```python
from build123d import *

# Parameters (mm, degrees)
BOSS_EXTRUDE1_DEPTH = 31.75
CUT_EXTRUDE1_DEPTH  = 25.4
FILLET1_R           = 2.54
CUT_EXTRUDE2_DEPTH  = 25.4
SKETCH5_R           = 0.762
CUT_EXTRUDE3_DEPTH  = 266.7


with BuildPart() as part:
    # Sketch1 → Boss-Extrude1 (new body)
    with BuildSketch(Plane(origin=(0, 0, 0), x_dir=(1, 0, 0), z_dir=(0, 1, 0))):
        with BuildLine():
            Line((12.429156122, 80.324059149), (20.977980966, 99.410685113))
            ThreePointArc((20.977980966, 99.410685113), (0, 101.6), (-20.977980966, 99.410685113))
            Line((-20.977980966, 99.410685113), (-12.429156122, 80.324059149))
            ThreePointArc((-12.429156122, 80.324059149), (0, 81.28), (12.429156122, 80.324059149))
        make_face()
    extrude(amount=BOSS_EXTRUDE1_DEPTH)

    # Sketch3 → Cut-Extrude1 (cut)
    with BuildSketch(Plane.XZ):
        with BuildLine():
            Line((-14.041319773, -83.923473707), (-15.916003555, -88.109006667))
            ThreePointArc((-15.916003555, -88.109006667), (0, -89.535), (15.916003555, -88.109006667))
            Line((15.916003555, -88.109006667), (14.041319773, -83.923473707))
            ThreePointArc((14.041319773, -83.923473707), (0, -85.09), (-14.041319773, -83.923473707))
        make_face()
    extrude(amount=-CUT_EXTRUDE1_DEPTH, mode=Mode.SUBTRACT)

    # Fillet1
    fillet1_edges = [part.edges().sort_by_distance(p)[0] for p in [
        (0, 31.75, -81.28),
        (0, 31.75, -101.6),
    ]]
    fillet(fillet1_edges, radius=FILLET1_R)

    # Sketch4 → Cut-Extrude2 (cut)
    with BuildSketch(Plane.XZ):
        with BuildLine():
            Line((-25.786806636, -94.723734325), (-24.259006715, -92.10897401))
            ThreePointArc((-24.259006715, -92.10897401), (10.833808817, -94.63187141), (44.448447191, -84.243088988))
            Line((44.448447191, -84.243088988), (46.527666616, -86.444904305))
            ThreePointArc((46.527666616, -86.444904305), (11.166045621, -97.533915466), (-25.786806636, -94.723734325))
        make_face()
    extrude(amount=-CUT_EXTRUDE2_DEPTH, mode=Mode.SUBTRACT)

    # Sketch5 → Cut-Extrude3 (cut)
    with BuildSketch(Plane.XY):
        with Locations((0, 6.35)):
            Circle(SKETCH5_R)
    extrude(amount=-CUT_EXTRUDE3_DEPTH, mode=Mode.SUBTRACT)


solid = part.part
```
Here's how the part is built. I have some questions about the finished solid (model axes, mm). A direction names the side the tool comes from. Round coordinates to 2 decimals unless told otherwise and drop trailing zeros. Order: outer loops, then holes, each group sorted by start corner. A loop starts at its lowest first (then second) coordinate and runs counter-clockwise, first axis right, second up. Notation, with made-up numbers: M 4.25,-19 L 24.25,-19 A20 cw 24.25,15 Z; hole C 60,-28 d8. An arc over 180 degrees is marked long. Answer as CSV lines item,"result".
Item 1: For pin 1 (1.5 mm diameter, centred on y = 24, z = -84.5, fed in from +X); pin 2 (2.5 mm diameter, centred on x = 0, y = 6.35, fed in from +Z); pin 3 (2 mm diameter, centred on x = 14.5, z = -86, fed in from -Y), each with a flat end and sliding along its axis, tell me the tip position at first contact or that it passes through.
From the geometry:
pin 1,"x = 14.04"
pin 2,"z = -81.27"
pin 3,"y = 25.4"
Item 2: Imagine slicing it at C-C on y = 6.35. List the corners of the cut face in (x, z) for me (3 decimals).
From the geometry:
outline,"M -20.978,-99.411 A101.6 ccw -0.762,-101.597 L -0.762,-98.168 A98.171 cw -19.543,-96.206 Z; M -18.318,-93.472 A95.25 ccw -0.762,-95.247 L -0.762,-89.532 A89.535 cw -15.916,-88.109 Z; M -14.041,-83.923 A85.09 ccw -0.762,-85.087 L -0.762,-81.276 A81.28 cw -12.429,-80.324 Z; M 0.762,-101.597 A101.6 ccw 20.978,-99.411 L 19.543,-96.206 A98.171 cw 0.762,-98.168 Z; M 0.762,-95.247 A95.25 ccw 18.318,-93.472 L 15.916,-88.109 A89.535 cw 0.762,-89.532 Z; M 0.762,-85.087 A85.09 ccw 14.041,-83.923 L 12.429,-80.324 A81.28 cw 0.762,-81.276 Z"
Item 3: Please list where these lines run through material, in increasing order: L1, parallel to Z at x = -1, y = 16; L2, parallel to Z at x = -11.5, y = 13; L3, parallel to Y at x = 0, z = -84.25. Write a range as [from, to].
From the geometry:
L1,"[-101.6, -98.17], [-95.24, -89.53], [-85.08, -81.27]"
L2,"[-100.95, -97.5], [-94.55, -88.79], [-84.31, -80.46]"
L3,"[0, 5.59], [7.11, 31.75]"
Item 4: Which directions (+Z, -Z, +X, -X, +Y, -Y) give clear straight access to the entire face, cutting with the end or side of a thin tool? Please do faces 1 (the cylindrical face through (0.4, 7, -83.2)), 2 (the cylindrical face through (0.2, 12.52, -85.09)).
From the geometry:
face 1,"+Z, -Z"
face 2,"-Y"
Item 5: Imagine slicing it at D-D on z = -91. List the corners of the cut face in (x, y) for me.
From the geometry:
outline,"M -17.21,0 L 17.21,0 L 17.21,31.75 L -17.21,31.75 Z; hole C 0,6.35 d1.52"
Item 6: We'd pull the mould along Z, two halves only. Please class faces 3 (the cylindrical face through (-0.17, 14.4, -81.28)), 4 (the cylindrical face through (-0.224, 12.522, -89.535)), 5 (the cylindrical face through (0.3, 14.4, -101.6)): +Z half, -Z half, draft (parallel to the pull), parting line (faces both ways), or undercut.
From the geometry:
face 3,"+Z half"
face 4,"undercut"
face 5,"-Z half"
Item 7: Imagine slicing it at B-B on y = 10.5. List the corners of the cut face in (x, z) for me (3 decimals), and give its area (3 significant figures).
From the geometry:
outline,"M -20.978,-99.411 A101.6 ccw 20.978,-99.411 L 19.543,-96.206 A98.171 cw -19.543,-96.206 Z; M -18.318,-93.472 A95.25 ccw 18.318,-93.472 L 15.916,-88.109 A89.535 cw -15.916,-88.109 Z; M -14.041,-83.923 A85.09 ccw 14.041,-83.923 L 12.429,-80.324 A81.28 cw -12.429,-80.324 Z"
area,"438 mm2"
Item 8: Imagine slicing it at A-A on x = 0. List the corners of the cut face in (y, z) for me (3 decimals), and give its area (3 significant figures).
From the geometry:
outline,"M 0,-101.6 L 5.588,-101.6 L 5.588,-98.171 L 0,-98.171 Z; M 0,-95.25 L 5.588,-95.25 L 5.588,-89.535 L 0,-89.535 Z; M 0,-85.09 L 5.588,-85.09 L 5.588,-81.28 L 0,-81.28 Z; M 7.112,-101.6 L 29.21,-101.6 A2.54 ccw 31.75,-99.06 L 31.75,-83.82 A2.54 ccw 29.21,-81.28 L 7.112,-81.28 L 7.112,-85.09 L 25.4,-85.09 L 25.4,-89.535 L 7.112,-89.535 L 7.112,-95.25 L 25.4,-95.25 L 25.4,-98.171 L 7.112,-98.171 Z"
area,"436 mm2"
